Read the model definition and answer for the solid it produces. Units are mm, in the model's axes. Give positions to 0.01 mm unless a question says otherwise; leave off trailing zeros. Order: outer loops, then holes, each group sorted by start corner. A loop starts at its lowest first (then second) coordinate and runs counter-clockwise, first axis right, second up. Notation, with made-up numbers: (80.25, 0.25) - (120.25, 0.25) arc R13 ccw to (120.25, 18.25) - close; hole circle Ø11 at (76.25, -36). An arc over 180 degrees is marked (long way). Write each question's results on one line, items separated by ' | '.
from build123d import *

# Parameters (mm, degrees)
EXTRUDE_1_DEPTH     = 5
SKETCH_2_W          = 20
SKETCH_2_H          = 3
SKETCH_2_W_2        = 10
SKETCH_2_H_2        = 30
SKETCH_2_H_3        = 50
CUT_EXTRUDE_1_DEPTH = 211.35683968
EXTRUDE_2_DEPTH     = 5
SKETCH_4_R          = 2
CUT_EXTRUDE_2_DEPTH = 620.212910153
SKETCH_6_W          = 3
SKETCH_6_H          = 50
SKETCH_6_H_2        = 104
EXTRUDE_3_DEPTH     = 5
EXTRUDE_4_DEPTH     = 5
SKETCH_8_R          = 2
SKETCH_8_W          = 50
SKETCH_8_H          = 10
CUT_EXTRUDE_3_DEPTH = 620.212910153
SKETCH_9_R          = 2
CUT_EXTRUDE_4_DEPTH = 620.212910153
SKETCH_10_R         = 7.5
CUT_EXTRUDE_5_DEPTH = 620.212910153
EXTRUDE_5_DEPTH     = 5
SKETCH_12_W         = 370.436309817
SKETCH_12_H         = 460
CUT_EXTRUDE_6_DEPTH = 641.99462376
SKETCH_15_R         = 2.5
SKETCH_15_R_2       = 12.5
CUT_EXTRUDE_7_DEPTH = 358.41919309
SKETCH_16_R         = 2
EXTRUDE_6_DEPTH     = 5


with BuildPart() as part:
    # 스케치1 → 보스-돌출1 (new body)
    with BuildSketch(Plane(origin=(0, 0, 0), x_dir=(1, 0, 0), z_dir=(0, 1, 0))):
        Polygon((-50, 175), (0, 175), (0, 185), (50, 185), (50, 175), (100, 175), (100, -175), (50, -175), (50, -185), (0, -185), (0, -175), (-50, -175), (-50, -185), (-100, -185), (-100, -175), (-100, 175), (-100, 185), (-50, 185), align=None)
    extrude(amount=EXTRUDE_1_DEPTH)

    # 스케치2 → 컷-돌출1 (cut, through all)
    with BuildSketch(Plane(origin=(0, 5, 0), x_dir=(1, 0, 0), z_dir=(0, 1, 0))):
        with Locations((70, 153.5)):
            Rectangle(SKETCH_2_W, SKETCH_2_H)
        with Locations((70, -153.5)):
            Rectangle(SKETCH_2_W, SKETCH_2_H)
        with Locations((45, 120)):
            Rectangle(SKETCH_2_W_2, SKETCH_2_H_2)
        with Locations((45, -120)):
            Rectangle(SKETCH_2_W_2, SKETCH_2_H_2)
        with Locations((45, 0)):
            Rectangle(SKETCH_2_W_2, SKETCH_2_H_3)
    extrude(amount=-CUT_EXTRUDE_1_DEPTH, mode=Mode.SUBTRACT)

    # 스케치3 → 보스-돌출2 (add)
    with BuildSketch(Plane(origin=(0, 5, 0), x_dir=(1, 0, 0), z_dir=(0, 1, 0))):
        Polygon((-540.91, 50), (-225, 50), (-100, 50), (-100, -50), (-225, -50), (-540.91, -50), (-540.91, -185), (-590.91, -185), (-590.91, 185), (-540.91, 185), align=None)
    extrude(amount=-EXTRUDE_2_DEPTH)

    # 스케치4 → 컷-돌출2 (cut, through all)
    with BuildSketch(Plane(origin=(0, 5, 0), x_dir=(1, 0, 0), z_dir=(0, 1, 0))):
        with Locations(Location((-578.91, 145, 0), (0, 0, 270))):
            Circle(SKETCH_4_R)
        with Locations(Location((-578.91, 95, 0), (0, 0, 270))):
            Circle(SKETCH_4_R)
        with Locations(Location((-566.91, 145, 0), (0, 0, 270))):
            Circle(SKETCH_4_R)
        with Locations(Location((-566.91, 95, 0), (0, 0, 270))):
            Circle(SKETCH_4_R)
        with Locations(Location((-578.91, -145, 0), (0, 0, 270))):
            Circle(SKETCH_4_R)
        with Locations(Location((-578.91, -95, 0), (0, 0, 270))):
            Circle(SKETCH_4_R)
        with Locations(Location((-566.91, -95, 0), (0, 0, 270))):
            Circle(SKETCH_4_R)
        with Locations(Location((-566.91, -145, 0), (0, 0, 270))):
            Circle(SKETCH_4_R)
    extrude(amount=-CUT_EXTRUDE_2_DEPTH, mode=Mode.SUBTRACT)

    # 스케치6 → 보스-돌출3 (add)
    with BuildSketch(Plane(origin=(0, 5, 0), x_dir=(1, 0, 0), z_dir=(0, 1, 0))):
        with Locations((101.5, -127)):
            Rectangle(SKETCH_6_W, SKETCH_6_H)
        with Locations((101.5, 127)):
            Rectangle(SKETCH_6_W, SKETCH_6_H)
        with Locations((101.5, 0)):
            Rectangle(SKETCH_6_W, SKETCH_6_H_2)
    extrude(amount=-EXTRUDE_3_DEPTH)

    # 스케치7 → 보스-돌출4 (add)
    with BuildSketch(Plane(origin=(0, 5, 0), x_dir=(1, 0, 0), z_dir=(0, 1, 0))):
        Polygon((-540.91, -185), (-537.91, -185), (-537.91, -92), (-495.91, -50), (-540.91, -50), align=None)
        Polygon((-537.91, 92), (-495.91, 50), (-540.91, 50), (-540.91, 185), (-537.91, 185), align=None)
        Polygon((-100, 95), (-145, 50), (-100, 50), align=None)
        Polygon((-100, -95), (-145, -50), (-100, -50), align=None)
    extrude(amount=-EXTRUDE_4_DEPTH)

    # 스케치8 → 컷-돌출3 (cut, through all)
    with BuildSketch(Plane(origin=(0, 5, 0), x_dir=(1, 0, 0), z_dir=(0, 1, 0))):
        with Locations(Location((-52, 86, 0), (0, 0, 270))):
            Circle(SKETCH_8_R)
        with Locations(Location((-52, 64, 0), (0, 0, 270))):
            Circle(SKETCH_8_R)
        with Locations(Location((26, 86, 0), (0, 0, 270))):
            Circle(SKETCH_8_R)
        with Locations(Location((26, 64, 0), (0, 0, 270))):
            Circle(SKETCH_8_R)
        with Locations(Location((-52, -86, 0), (0, 0, 90))):
            Circle(SKETCH_8_R)
        with Locations(Location((-52, -64, 0), (0, 0, 90))):
            Circle(SKETCH_8_R)
        with Locations(Location((26, -64, 0), (0, 0, 90))):
            Circle(SKETCH_8_R)
        with Locations(Location((26, -86, 0), (0, 0, 90))):
            Circle(SKETCH_8_R)
        with Locations((-13, 75)):
            Rectangle(SKETCH_8_W, SKETCH_8_H)
        with Locations((-13, -75)):
            Rectangle(SKETCH_8_W, SKETCH_8_H)
    extrude(amount=-CUT_EXTRUDE_3_DEPTH, mode=Mode.SUBTRACT)

    # 스케치9 → 컷-돌출4 (cut, through all)
    with BuildSketch(Plane(origin=(0, 5, 0), x_dir=(1, 0, 0), z_dir=(0, 1, 0))):
        with Locations(Location((-437.91, 30, 0), (0, 0, 270))):
            Circle(SKETCH_9_R)
        with Locations(Location((-235.58, 30, 0), (0, 0, 270))):
            Circle(SKETCH_9_R)
        with Locations(Location((-185.58, 30, 0), (0, 0, 270))):
            Circle(SKETCH_9_R)
        with Locations(Location((-185.58, -30, 0), (0, 0, 90))):
            Circle(SKETCH_9_R)
        with Locations(Location((-235.58, -30, 0), (0, 0, 90))):
            Circle(SKETCH_9_R)
        with Locations(Location((-437.91, -30, 0), (0, 0, 90))):
            Circle(SKETCH_9_R)
    extrude(amount=-CUT_EXTRUDE_4_DEPTH, mode=Mode.SUBTRACT)

    # 스케치10 → 컷-돌출5 (cut, through all)
    with BuildSketch(Plane(origin=(0, 5, 0), x_dir=(1, 0, 0), z_dir=(0, 1, 0))):
        with Locations(Location((-73, 0, 0), (0, 0, 270))):
            Circle(SKETCH_10_R)
    extrude(amount=-CUT_EXTRUDE_5_DEPTH, mode=Mode.SUBTRACT)

    # 스케치11 → 보스-돌출5 (add)
    with BuildSketch(Plane(origin=(0, 5, 0), x_dir=(1, 0, 0), z_dir=(0, 1, 0))):
        Polygon((-145, -50), (-257, -50), (-257, -248.343471002), (103, -248.343471002), (103, -152), (100, -152), (100, -175), (50, -175), (50, -185), (0, -185), (0, -175), (-50, -175), (-50, -185), (-100, -185), (-100, -95), align=None)
        Polygon((103, 152), (103, 211.656528998), (-257, 211.656528998), (-257, 50), (-145, 50), (-100, 95), (-100, 185), (-50, 185), (-50, 175), (0, 175), (0, 185), (50, 185), (50, 175), (100, 175), (100, 152), align=None)
    extrude(amount=-EXTRUDE_5_DEPTH)

    # 스케치12 → 컷-돌출6 (cut, through all)
    with BuildSketch(Plane(origin=(0, 5, 0), x_dir=(1, 0, 0), z_dir=(0, 1, 0))):
        with Locations((-442.218154909, -18.343471002)):
            Rectangle(SKETCH_12_W, SKETCH_12_H)
    extrude(amount=-CUT_EXTRUDE_6_DEPTH, mode=Mode.SUBTRACT)

    # 스케치15 → 컷-돌출7 (cut, through all)
    with BuildSketch(Plane(origin=(0, 5, 0), x_dir=(1, 0, 0), z_dir=(0, 1, 0))):
        with Locations(Location((-73.050208533, -55.416458765, 0), (0, 0, 270))):
            Circle(SKETCH_15_R)
        with Locations(Location((-128.050208533, -0.416458765, 0), (0, 0, 270))):
            Circle(SKETCH_15_R)
        with Locations(Location((-73.050208533, 54.583541235, 0), (0, 0, 270))):
            Circle(SKETCH_15_R)
        with Locations(Location((-18.050208533, -0.416458765, 0), (0, 0, 270))):
            Circle(SKETCH_15_R)
        with Locations(Location((-73.050208533, -0.416458765, 0), (0, 0, 270))):
            Circle(SKETCH_15_R_2)
        with Locations(Location((-242, 201.656528998, 0), (0, 0, 270))):
            Circle(SKETCH_15_R)
        with Locations(Location((-92, 201.656528998, 0), (0, 0, 270))):
            Circle(SKETCH_15_R)
        with Locations(Location((78, 201.656528998, 0), (0, 0, 270))):
            Circle(SKETCH_15_R)
        with Locations(Location((78, -238.343471002, 0), (0, 0, 90))):
            Circle(SKETCH_15_R)
        with Locations(Location((-92, -238.343471002, 0), (0, 0, 90))):
            Circle(SKETCH_15_R)
        with Locations(Location((-242, -238.343471002, 0), (0, 0, 90))):
            Circle(SKETCH_15_R)
    extrude(amount=-CUT_EXTRUDE_7_DEPTH, mode=Mode.SUBTRACT)

    # 스케치16 → 보스-돌출6 (add)
    with BuildSketch(Plane(origin=(0, 5, 0), x_dir=(1, 0, 0), z_dir=(0, 1, 0))):
        with Locations((-185.58, -30)):
            Circle(SKETCH_16_R)
        with Locations((-235.58, -30)):
            Circle(SKETCH_16_R)
        with Locations((-185.58, 30)):
            Circle(SKETCH_16_R)
        with Locations((-235.58, 30)):
            Circle(SKETCH_16_R)
    extrude(amount=-EXTRUDE_6_DEPTH)


solid = part.part
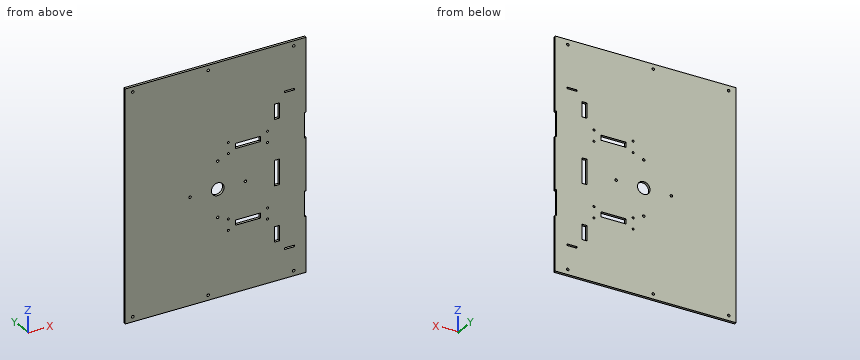
(1) This flat-tipped pin is pushed along its axis until it touches: pin 1 (6 mm diameter, centred on x = -92, z = -201.66, fed in from -Y). Where does it stop, or does it pass through?
Conclusion:
pin 1: y = 0
(2) Consider probe 1 along Z at (x, y) = (-7, 3.45); probe 2 along X at (y, z) = (3.6, 86); probe 3 along Z at (x, y) = (-51.5, 2.75). Determine where each line is inside the solid, lowest interval first. Write a range as [from, to].
Conclusion:
probe 1: [-211.66, -80], [-70, 70], [80, 248.34] | probe 2: [-257, -54], [-50, 24], [28, 100] | probe 3: [-211.66, -87.94], [-84.06, -65.94], [-62.06, 62.06], [65.94, 84.06], [87.94, 248.34]
(3) Section A-A (x = -6.5) is taken. Give the vertices of the cut face in (y, z), plus the area to 3 significant figures.
Conclusion:
outline: (0, -211.66) - (5, -211.66) - (5, -80) - (0, -80) - close; (0, -70) - (5, -70) - (5, 70) - (0, 70) - close; (0, 80) - (5, 80) - (5, 248.34) - (0, 248.34) - close | area: 2,200 mm^2
(4) Section B-B (y = 3) is taken. State how many separate pieces and enclosed holes the cut face has, plus the area to 3 significant figures.
Conclusion:
separate pieces: 1 | enclosed holes: 26 | area: 162,000 mm^2
